from build123d import *

# Parameters (mm, degrees)
IZIM1_R                     = 2.6
Y_KSEKLIK_EKSTR_ZYON1_DEPTH = 7
IZIM3_R                     = 11.25
IZIM3_R_2                   = 8
Y_KSEKLIK_EKSTR_ZYON2_DEPTH = 20
KES_EKSTR_ZYON1_DEPTH       = 40
KES_EKSTR_ZYON1_DEPTH_BACK  = 5
IZIM4_R                     = 9
RADYUS2_R                   = 6


with BuildPart() as part:
    # Çizim1 → Yükseklik-Ekstrüzyon1 (new body)
    with BuildSketch(Plane(origin=(0, 0, 0), x_dir=(1, 0, 0), z_dir=(0, 1, 0))):
        with BuildLine():
            Line((-31.166666667, 6.236095645), (-12.5, 18.708286934))
            ThreePointArc((-12.5, 18.708286934), (0, 22.5), (12.5, 18.708286934))
            Line((12.5, 18.708286934), (31.166666667, 6.236095645))
            ThreePointArc((31.166666667, 6.236095645), (34.5, 0), (31.166666667, -6.236095645))
            Line((31.166666667, -6.236095645), (12.5, -18.708286934))
            ThreePointArc((12.5, -18.708286934), (0, -22.5), (-12.5, -18.708286934))
            Line((-12.5, -18.708286934), (-31.166666667, -6.236095645))
            ThreePointArc((-31.166666667, -6.236095645), (-34.5, 0), (-31.166666667, 6.236095645))
        make_face()
        with Locations(Location((-27, 0, 0), (0, 0, 270))):
            Circle(IZIM1_R, mode=Mode.SUBTRACT)
        with Locations(Location((27, 0, 0), (0, 0, 270))):
            Circle(IZIM1_R, mode=Mode.SUBTRACT)
    extrude(amount=Y_KSEKLIK_EKSTR_ZYON1_DEPTH)

    # Çizim3 → Yükseklik-Ekstrüzyon2 (add)
    with BuildSketch(Plane(origin=(0, 7, 0), x_dir=(1, 0, 0), z_dir=(0, 1, 0))):
        with Locations(Location((0, 0, 0), (0, 0, 270))):
            Circle(IZIM3_R)
        with Locations(Location((0, 0, 0), (0, 0, 270))):
            Circle(IZIM3_R_2, mode=Mode.SUBTRACT)
    extrude(amount=Y_KSEKLIK_EKSTR_ZYON2_DEPTH)

    # Çizim4 → Kes-Ekstrüzyon1 (cut, two sides: drawn at the far end of the back side and taken through both)
    with BuildSketch(Plane(origin=(0, 7, 0), x_dir=(1, 0, 0), z_dir=(0, 1, 0)).offset(-KES_EKSTR_ZYON1_DEPTH_BACK)):
        with Locations(Location((0, 0, 0), (0, 0, 90))):
            Circle(IZIM4_R)
    extrude(amount=KES_EKSTR_ZYON1_DEPTH + KES_EKSTR_ZYON1_DEPTH_BACK, mode=Mode.SUBTRACT)

    # Radyus2
    radyus2_edges = [part.edges().sort_by_distance(p)[0] for p in [
        (0, 7, -11.25),
    ]]
    fillet(radyus2_edges, radius=RADYUS2_R)


solid = part.part
Model file for the job. Use its own axes, mm. A direction names the side the tool comes from. Round coordinates to 2 decimals unless told otherwise and drop trailing zeros. Loops run counter-clockwise (first coordinate to the right, second up) from the corner with the lowest first, then second, coordinate; pieces in that order, holes last. Notation, with made-up numbers: (47, -28.5) -> (84, -28.5) arc R10 cw to (84, -10.5) -> close; hole circle Ø11 at (-35, 23.5). An arc over 180 degrees is marked (long way). Answer as CSV lines item,"result". Start each with the question number.
1) Slice it at B-B (y = 3.75). List the corners of the cut face in (x, z).
2) Tool access for faces 4 (the face through (21.7, 3.45, -12.56)), 5 (the face through (0, 2, 0)): list every direction of +Z, -Z, +X, -X, +Y, -Y with a clear straight run to the whole face (end or side of a thin tool).
3) Probe line 1 along Y through (x, z) = (17.5, 7.5); line 2 along X through (y, z) = (17.75, 0); line 3 along Z through (x, y) = (-7, 15.5). List the from-to ranges inside material, lowest first.
4) Slice it at C-C (x = -27). List the corners of the cut face in (y, z), plus the area to 3 significant figures.
5) Slice it at A-A (z = 0). List the corners of the cut face in (x, y), plus the area to 3 significant figures.
6) Mould opens along Z. For faces 1 (the face through (8, 27, -5)), 2 (the face through (-34.5, 3.5, 0.1)), 3 (the face through (-2.703, 14.325, -8.584)) say: +Z half, -Z half, draft (parallel to the pull), parting line (faces both ways), or undercut.
7) Pin check, flat tips, straight feed: P1, Ø5, axis at x = 4.5, y = 18, coming from the -Z side; P2, Ø6, axis at y = 7, z = -5.5, coming from the -X side; P3, Ø2, axis at y = 11.5, z = -2.5, coming from the +X side. Stop position of each tip, or through.
8) Slice it at D-D (x = 0). List the corners of the cut face in (y, z).
Filled in:
1,outline,"(-31.17, -6.24) -> (-12.5, -18.71) arc R22.5 ccw to (12.5, -18.71) -> (31.17, -6.24) arc R7.5 ccw to (31.17, 6.24) -> (12.5, 18.71) arc R22.5 ccw to (-12.5, 18.71) -> (-31.17, 6.24) arc R7.5 ccw to start; hole circle Ø5.2 at (-27, 0); hole circle Ø18 at (0, 0); hole circle Ø5.2 at (27, 0)"
2,face 4,"-Z, +X, +Y, -Y"
2,face 5,"+Y"
3,line 1,"y = 0 to 7"
3,line 2,"x = -11.25 to -9, 9 to 11.25"
3,line 3,"z = -8.81 to -5.66, 5.66 to 8.81"
4,outline,"(0, -9.02) -> (7, -9.02) -> (7, -2.6) -> (0, -2.6) -> close; (0, 2.6) -> (7, 2.6) -> (7, 9.02) -> (0, 9.02) -> close"
4,area,"89.9 mm2"
5,outline,"(-34.5, 0) -> (-29.6, 0) -> (-29.6, 7) -> (-34.5, 7) -> close; (-24.4, 0) -> (24.4, 0) -> (24.4, 7) -> (17.25, 7) arc R6 cw to (11.25, 13) -> (11.25, 27) -> (9, 27) -> (9, 2) -> (-9, 2) -> (-9, 27) -> (-11.25, 27) -> (-11.25, 13) arc R6 cw to (-17.25, 7) -> (-24.4, 7) -> close; (29.6, 0) -> (34.5, 0) -> (34.5, 7) -> (29.6, 7) -> close"
5,area,"426 mm2"
6,face 1,"draft"
6,face 2,"parting line"
6,face 3,"undercut"
7,P1,"stops at z = -11.07"
7,P2,"stops at x = -34.07"
7,P3,"stops at x = 11.57"
8,outline,"(0, -22.5) -> (7, -22.5) -> (7, -17.25) arc R6 cw to (13, -11.25) -> (27, -11.25) -> (27, -9) -> (2, -9) -> (2, 9) -> (27, 9) -> (27, 11.25) -> (13, 11.25) arc R6 cw to (7, 17.25) -> (7, 22.5) -> (0, 22.5) -> close"
